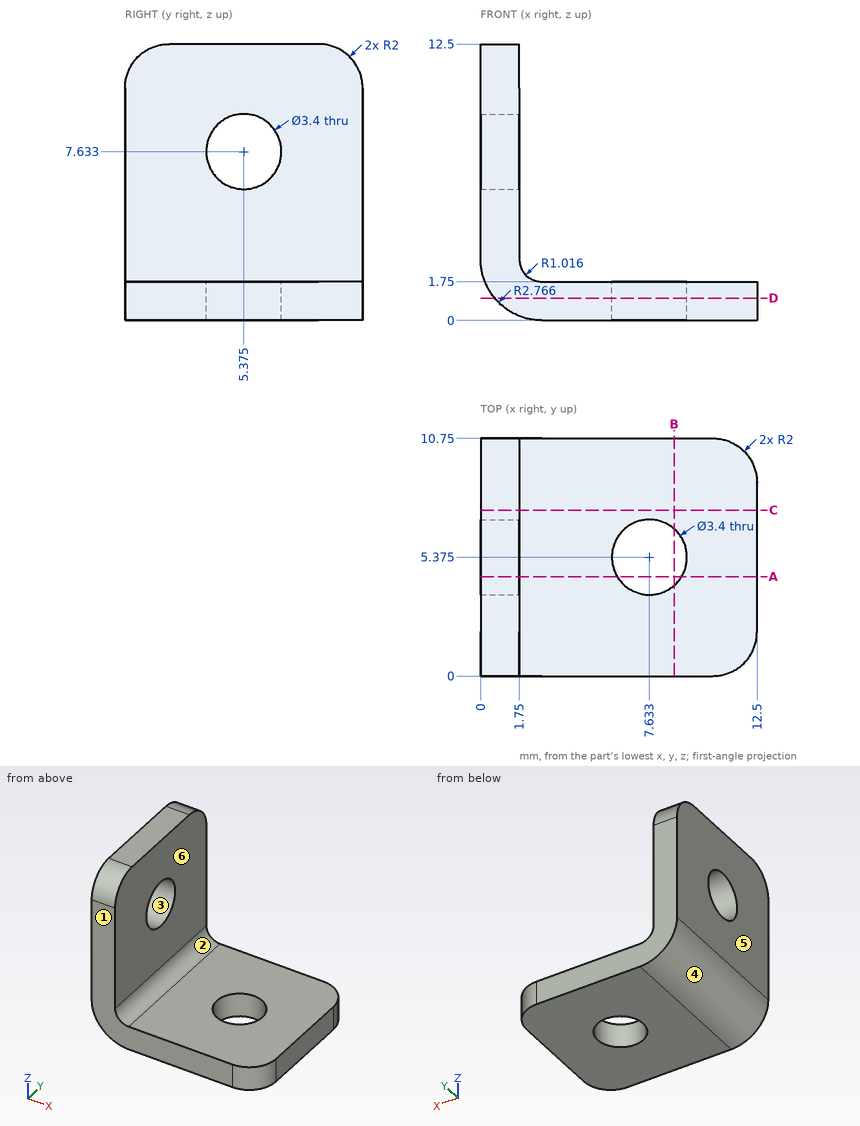
Geometry check sheet. Reference: drawing and pictorial views, mm from the part's lowest x, y, z. A direction names the side the tool comes from. Coordinates: 2 decimals unless noted, no trailing zeros. Order: outer loops, then holes, each group sorted by start corner. A loop starts at its lowest first (then second) coordinate and runs counter-clockwise, first axis right, second up. Notation, with made-up numbers: (89.25, 28.5) - (107.25, 28.5) arc R4 cw to (107.25, 34.5) - close; hole circle Ø3 at (3, 88.25). An arc over 180 degrees is marked (long way). Answer in a Markdown table with one row per item. Add a question column.
1) Release check for a two-part mould opening along Z. For the marked faces 1, 2, 3 and 4 record: +Z half, -Z half, draft (parallel to the pull), parting line (faces both ways), or undercut.
2) Set-up check for the marked faces 5 and 6: record each of +Z, -Z, +X, -X, +Y, -Y from which the full face is reachable in a straight line by a thin tool's end or side.
3) Cross-section at C-C, the plane y = 7.5. Record the cut outline in (x, z).
4) Cross-section at D-D, the plane z = 1. Record the cut outline in (x, y) (3 decimals), then the cut area to 3 significant figures.
5) Gauge pin test, flat ends, axial feed: P1, Ø5.5, axis at x = 7.633, y = 5.375, coming from the -Z side; P2, Ø4, axis at x = 7, y = 8.5, coming from the +Z side; P3, Ø4, axis at x = 4.5, z = 11, coming from the -Y side; P4, Ø4, axis at y = 2.5, z = 6, coming from the +X side. Record the tip position at first contact, or that the pin passes through.
6) Cross-section at A-A, the plane y = 4.5. Record the cut outline in (x, z), then the cut area to 3 significant figures.
7) Material ranges on line 1 along Z through (x, y) = (4.25, 5); line 2 along X through (y, z) = (9.5, 0.75), recorded low to high. Write a range as [from, to].
8) Cross-section at B-B, the plane x = 8.75. Record the cut outline in (y, z), then the cut area to 3 significant figures.
Check result:
| question | item | result |
|---|---|---|
| 1 | face 1 | draft |
| 1 | face 2 | +Z half |
| 1 | face 3 | undercut |
| 1 | face 4 | -Z half |
| 2 | face 5 | +Z, -Z, -X, +Y, -Y |
| 2 | face 6 | +Z, +X, +Y, -Y |
| 3 | outline | (0, 2.77) arc R2.77 ccw to (2.77, 0) - (12.5, 0) - (12.5, 1.75) - (2.77, 1.75) arc R1.02 cw to (1.75, 2.77) - (1.75, 12.5) - (0, 12.5) - close |
| 4 | outline | (0.637, 0) - (10.5, 0) arc R2 ccw to (12.5, 2) - (12.5, 8.75) arc R2 ccw to (10.5, 10.75) - (0.637, 10.75) - close; hole circle Ø3.4 at (7.633, 5.375) |
| 4 | area | 117 mm² |
| 5 | P1 | stops at z = 0 |
| 5 | P2 | stops at z = 1.75 |
| 5 | P3 | passes through |
| 5 | P4 | stops at x = 1.75 |
| 6 | outline | (0, 2.77) arc R2.77 ccw to (2.77, 0) - (6.18, 0) - (6.18, 1.75) - (2.77, 1.75) arc R1.02 cw to (1.75, 2.77) - (1.75, 6.18) - (0, 6.18) - close; (0, 9.09) - (1.75, 9.09) - (1.75, 12.5) - (0, 12.5) - close; (9.09, 0) - (12.5, 0) - (12.5, 1.75) - (9.09, 1.75) - close |
| 6 | area | 29.1 mm² |
| 7 | line 1 | z = [0, 1.75] |
| 7 | line 2 | x = [0.87, 12.35] |
| 8 | outline | (0, 0) - (4.09, 0) - (4.09, 1.75) - (0, 1.75) - close; (6.66, 0) - (10.75, 0) - (10.75, 1.75) - (6.66, 1.75) - close |
| 8 | area | 14.3 mm² |
